Autodesk Inventor part; units mm, degrees
ref_plane "YZ Plane" through (0, 0, 0) normal (1, 0, 0) x (0, 1, 0)
ref_plane "XZ Plane" through (0, 0, 0) normal (0, 1, 0) x (-1, 0, 0)
ref_plane "XY Plane" through (0, 0, 0) normal (0, 0, 1) x (1, 0, 0)
sketch "Sketch1" plane through (0, 0, 0) normal (0, 0, 1) x (1, 0, 0)
  line L0 (50, -5) -> (50, 23)
  line L1 (50, 23) -> (8, 23)
  line L2 (18, 10) -> (38, 10)
  line L3 (18, 10) -> (18, -5)
  line L4 (38, 10) -> (38, -5)
  line L5 (8, -5) -> (8, 23)
  line L6 (8, -5) -> (18, -5)
  line L7 (38, -5) -> (50, -5)
  dimension "d1" = 28
  dimension "d4" = 15
  dimension "d14" = 20
  dimension "d16" = 12
  dimension "d37" = 42
  dimension "d46" = 28
extrude "Extrusion3" add sketch "Sketch1" along normal blind 10
sketch "Sketch5" plane through (8, -5, 0) normal (0, -1, 0) x (1, 0, 0)
  circle A0 centre (4, 5) radius 2
  line L0 (10, 0) -> (10, 10)
  line L1 (0, 0) -> (10, 0)
  circle A1 centre (36, 5) radius 2
  line L2 (30, 0) -> (30, 10)
  line L3 (30, 0) -> (42, 0)
  dimension "d38" = 4
  dimension "d39" = 6
  dimension "d40" = 5
  dimension "d41" = 4
  dimension "d42" = 6
  dimension "d43" = 5
extrude "Extrusion6" cut sketch "Sketch5" against normal blind 100
sketch "Boceto6" plane through (0, 0, 10) normal (0, 0, 1) x (1, 0, 0)
  line L0 (50, 23) -> (8, 23)
  circle A0 centre (23, 13) radius 1.5
  circle A1 centre (33, 13) radius 1.5
  line L1 (50, -5) -> (50, 23)
  line L2 (38, 10) -> (38, -5)
  point P0 (0, 0)
  dimension "d50" = 3
  dimension "d51" = 3
  dimension "d52" = 10
  dimension "d53" = 10
  dimension "d62" = 5
extrude "Extrusión7" cut sketch "Boceto6" against normal blind 10
thread "Rosca1"
thread "Rosca2"
properties part number "Espaciador Izquierdo" material "Aluminum 6061"
Read the model definition and answer for the solid it produces. Units are mm, in the model's axes. A direction names the side the tool comes from. Round coordinates to 2 decimals unless told otherwise and drop trailing zeros. Order: outer loops, then holes, each group sorted by start corner. A loop starts at its lowest first (then second) coordinate and runs counter-clockwise, first axis right, second up.
1) A flat-ended cylindrical pin translates along its axis: pin 1 (5 mm diameter, centred on x = 30.5, z = 2, fed in from -Y). Find the tip coordinate at first contact, or state that the pin passes through.
2) Straight lines are drawn through the part: L1, parallel to Y at x = 23, z = 6.75; L2, parallel to X at y = 6.75, z = 2; L3, parallel to Z at x = 44, y = 5.5. For each, find the intervals that lie inside material, in ascending order.
3) The part is cut by section A-A on y = -0.25. Write down the section's boundary in (x, z), plus the area to 3 significant figures.
4) The part is cut by section C-C on x = 23. Write down the section's boundary in (y, z), plus the area to 3 significant figures.
5) For faces 1 (the face through (38, 3, 5)), 2 (the face through (43.9, -5, 2.7)), determine the directions among +Z, -Z, +X, -X, +Y, -Y from which every point of the face is accessible in a straight line to the end or side of a thin tool.
6) The part is cut by section D-D on y = 13. Write down the section's boundary in (x, z), plus the area to 3 significant figures.
7) The part is cut by section B-B on z = 5. Write down the section's boundary in (x, y), plus the area to 3 significant figures.
8) The mould has two halves that part along X. Classify faces 3 (the face through (50, 9, 5)), 4 (the face through (8, 9, 5)), 5 (the face through (31.5, 13.07, 5.07)), 6 (the face through (29, 12, 0)): released by +X, released by -X, zero draft, split by the parting line, or undercut.
Resolved:
1. pin 1: stops at y = 10
2. L1: y = 10 to 11.5, 14.5 to 23
2. L2: x = 8 to 18, 38 to 50
2. L3: z = 0 to 3, 7 to 10
3. outline: (8, 0) - (18, 0) - (18, 10) - (8, 10) - close; (38, 0) - (50, 0) - (50, 10) - (38, 10) - close; hole circle Ø4 at (12, 5); hole circle Ø4 at (44, 5)
3. area: 195 mm2
4. outline: (10, 0) - (11.5, 0) - (11.5, 10) - (10, 10) - close; (14.5, 0) - (23, 0) - (23, 10) - (14.5, 10) - close
4. area: 100 mm2
5. face 1: +Z, -Z, -Y
5. face 2: +Z, -Z, +X, -X, -Y
6. outline: (8, 0) - (21.5, 0) - (21.5, 10) - (8, 10) - close; (24.5, 0) - (31.5, 0) - (31.5, 10) - (24.5, 10) - close; (34.5, 0) - (50, 0) - (50, 10) - (34.5, 10) - close; hole circle Ø4 at (12, 5); hole circle Ø4 at (44, 5)
6. area: 335 mm2
7. outline: (8, -5) - (10, -5) - (10, 23) - (8, 23) - close; (14, -5) - (18, -5) - (18, 10) - (38, 10) - (38, -5) - (42, -5) - (42, 23) - (14, 23) - close; (46, -5) - (50, -5) - (50, 23) - (46, 23) - close; hole circle Ø3 at (23, 13); hole circle Ø3 at (33, 13)
7. area: 638 mm2
8. face 3: released by +X
8. face 4: released by -X
8. face 5: undercut
8. face 6: zero draft
